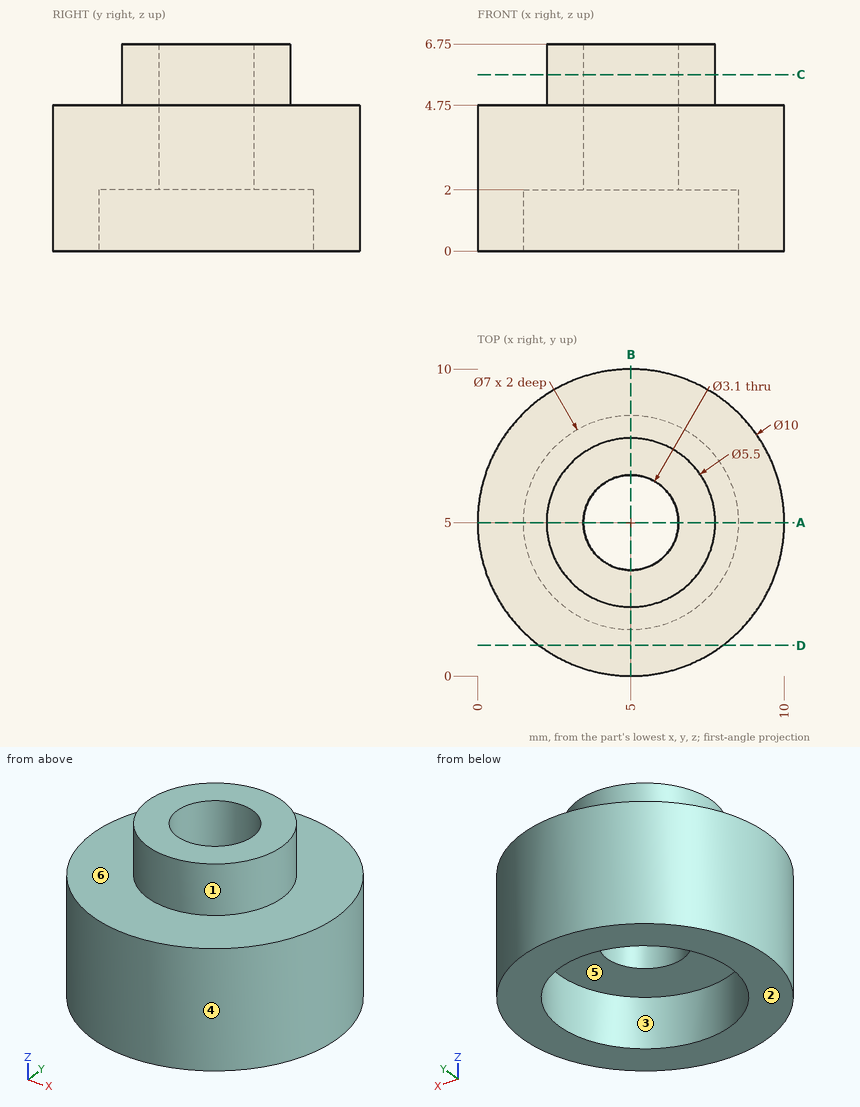
Check sheet for the drawn part. Datum: minimum x, y, z corner. Units: mm. A direction names the side the tool comes from. Give positions to 0.01 mm unless a question says otherwise; leave off trailing zeros. Order: outer loops, then holes, each group sorted by start corner. A loop starts at its lowest first (then second) coordinate and runs counter-clockwise, first axis right, second up. Notation, with made-up numbers: (27, 82) -> (47, 82) arc R25 cw to (47, 121) -> close; hole circle Ø11 at (48, -5.75). An arc over 180 degrees is marked (long way). Return JSON: item names as keys, results as strings.
1. Go/stop test with flat-tipped pins: P1, Ø4, axis at x = 8.5, z = 2.5, coming from the +Y side; P2, Ø4, axis at x = 5, y = 5, coming from the -Z side; P3, Ø5.5, axis at x = 5, y = 5, coming from the +Z side; P4, Ø1.5, axis at y = 2.5, z = 1, coming from the +X side. Record where each tip stops, or that it passes through.
From the geometry:
{"P1": "y = 9.77", "P2": "z = 2", "P3": "z = 6.75", "P4": "x = 9.68"}
2. Cross-section at C-C, the plane z = 5.75. Record the cut outline in (x, y).
From the geometry:
{"outline": "circle Ø5.5 at (5, 5); hole circle Ø3.1 at (5, 5)"}
3. Cross-section at A-A, the plane y = 5. Record the cut outline in (x, z).
From the geometry:
{"outline": "(0, 0) -> (1.5, 0) -> (1.5, 2) -> (3.45, 2) -> (3.45, 6.75) -> (2.25, 6.75) -> (2.25, 4.75) -> (0, 4.75) -> close; (6.55, 2) -> (8.5, 2) -> (8.5, 0) -> (10, 0) -> (10, 4.75) -> (7.75, 4.75) -> (7.75, 6.75) -> (6.55, 6.75) -> close"}
4. Cross-section at D-D, the plane y = 1. Record the cut outline in (x, z).
From the geometry:
{"outline": "(2, 0) -> (8, 0) -> (8, 4.75) -> (2, 4.75) -> close"}
5. Mould release check, pull along X, two halves, no side actions. Record for the marked faces 4, 5 and 6: +X half, -X half, draft (parallel to the pull), parting line (faces both ways), or undercut.
From the geometry:
{"face 4": "parting line", "face 5": "undercut", "face 6": "draft"}
6. Set-up check for the marked faces 1, 2 and 3: record each of +Z, -Z, +X, -X, +Y, -Y from which the full face is reachable in a straight line by a thin tool's end or side.
From the geometry:
{"face 1": "+Z", "face 2": "-Z, +X, -X, +Y, -Y", "face 3": "-Z"}
7. Material ranges on probe 1 along Y at (x, z) = (5, 5.8); probe 2 along Y at (x, z) = (5, 3.7); probe 3 along Z at (x, y) = (7, 4.25), recorded low to high. Write a range as [from, to].
From the geometry:
{"probe 1": "[2.25, 3.45], [6.55, 7.75]", "probe 2": "[0, 3.45], [6.55, 10]", "probe 3": "[2, 6.75]"}
